```python
from build123d import *

# Parameters (mm, degrees)
F0_W     = 60
F0_H     = 60
F1_DEPTH = 1.5
F2_R     = 3
F4_D     = 2.65


with BuildPart() as f1:
    # F0 (on Top) → F1 (new body)
    with BuildSketch(Plane.XY):
        Rectangle(F0_W, F0_H)
    extrude(amount=F1_DEPTH)

    # F2
    f2_edges = [f1.edges().sort_by_distance(p)[0] for p in [
        (-30, -30, 0.75),
        (30, -30, 0.75),
        (30, 30, 0.75),
        (-30, 30, 0.75),
    ]]
    fillet(f2_edges, radius=F2_R)

    # F4 (through all)
    with Locations(Plane.XY.offset(1.5)):
        with Locations((-15, 10), (15, 10), (15, -10), (-15, -10), (-8.9, 26.1), (19, 26.1), (24.1, -26), (-24.1, -24.7)):
            Hole(F4_D / 2)


solid = f1.part
```
The listing builds one solid part. Answer for the finished solid, in the listing's coordinates (mm). Coordinates: 2 decimals unless noted, no trailing zeros. Loops run counter-clockwise (first coordinate to the right, second up) from the corner with the lowest first, then second, coordinate; pieces in that order, holes last. Notation, with made-up numbers: (54.25, 89.5) -> (96.25, 89.5) arc R33 cw to (96.25, 121.5) -> close; hole circle Ø7 at (75.5, 25.25). An arc over 180 degrees is marked (long way). Use one line per item in the form item = value. Start each with the question number.
Item 1: The part is cut by section D-D on x = 19.5. Determine the outline of the cut face in (y, z).
Item 2: Consider L1, parallel to X at y = 11, z = 0.4; L2, parallel to Y at x = -24.5, z = 0.5; L3, parallel to Y at x = 19, z = 0.65 (3 decimals). Determine where each line is inside the solid, lowest interval first. Write a range as [from, to].
Item 3: The part is cut by section C-C on x = -24.1. Determine the outline of the cut face in (y, z) (3 decimals), then the cut area to 3 significant figures.
Item 4: The part is cut by section B-B on y = 26.1. Determine the outline of the cut face in (x, z) (3 decimals).
Item 5: The mould has two halves that part along X. Classify faces 1 (the face through (0, -30, 1)), 2 (the face through (-29.14, -29.1, 0.76)), 3 (the face through (16.324, 10.058, 0.74)): released by +X, released by -X, zero draft, split by the parting line, or undercut.
Item 6: A flat-ended cylindrical pin translates along its axis: pin 1 Ø2.5 at (x, y) = (-15, 10) entering from +Z (3 decimals). Find the tip coordinate at first contact, or state that the pin passes through.
Item 7: The part is cut by section A-A on x = -15. Determine the outline of the cut face in (y, z) (3 decimals).
Answer key:
q1.outline = (-30, 0) -> (24.87, 0) -> (24.87, 1.5) -> (-30, 1.5) -> close; (27.33, 0) -> (30, 0) -> (30, 1.5) -> (27.33, 1.5) -> close
q2.L1 = [-30, -15.87], [-14.13, 14.13], [15.87, 30]
q2.L2 = [-30, -25.96], [-23.44, 30]
q2.L3 = [-30, 24.775], [27.425, 30]
q3.outline = (-30, 0) -> (-26.025, 0) -> (-26.025, 1.5) -> (-30, 1.5) -> close; (-23.375, 0) -> (30, 0) -> (30, 1.5) -> (-23.375, 1.5) -> close
q3.area = 86.0 mm2
q4.outline = (-30, 0) -> (-10.225, 0) -> (-10.225, 1.5) -> (-30, 1.5) -> close; (-7.575, 0) -> (17.675, 0) -> (17.675, 1.5) -> (-7.575, 1.5) -> close; (20.325, 0) -> (30, 0) -> (30, 1.5) -> (20.325, 1.5) -> close
q5.face_1 = zero draft
q5.face_2 = released by -X
q5.face_3 = undercut
q6.pin_1 = through
q7.outline = (-30, 0) -> (-11.325, 0) -> (-11.325, 1.5) -> (-30, 1.5) -> close; (-8.675, 0) -> (8.675, 0) -> (8.675, 1.5) -> (-8.675, 1.5) -> close; (11.325, 0) -> (30, 0) -> (30, 1.5) -> (11.325, 1.5) -> close
